Part model, mm, in its own coordinate system. A direction names the side the tool comes from. Coordinates: 2 decimals unless noted, no trailing zeros. Loops run counter-clockwise (first coordinate to the right, second up) from the corner with the lowest first, then second, coordinate; pieces in that order, holes last. Notation, with made-up numbers: M 73,42.5 L 98,42.5 A20 ccw 98,65.5 Z; hole C 80,83.25 d7. An arc over 180 degrees is marked long. Use a Markdown table: item, result. Add a question column.
1) Band-saw the part on C-C (x = -22). List the corners of the cut face in (y, z) (1 decimal).
2) Pull direction X, two halves, no side cores. Call faces 1 (the flat face through (43.815, -4, 0)), 2 (the cylindrical face through (-26.5, -11.3, 0)), 3 (the flat face through (1, -14.288, 0)): released by +X, released by -X, zero draft, split by the parting line, or undercut.
3) Pin check, flat tips, straight feed: pin 1 Ø3 at (x, z) = (18, -2) entering from +Y; pin 2 Ø3 at (y, z) = (-5.5, 1) entering from +X (3 decimals); pin 3 Ø2 at (y, z) = (-4.5, -2) entering from -X (3 decimals). Stop position of each tip, or through.
4) Wall check: probe 1 along X at (y, z) = (-1.5, 2.5) (3 decimals); probe 2 along X at (y, z) = (-9.75, 0); probe 3 along X at (y, z) = (-5, -1.5) (3 decimals). Give the ranges that are in metal, low to high. Write a range as from..to.
5) Tool access for faces 4 (the cylindrical face through (-43.545, -13.333, 0.044)), 5 (the cylindrical face through (-39.25, -5.63, -0.04)), 6 (the flat face through (-40, -10, 1.905)): list every direction of +Z, -Z, +X, -X, +Y, -Y with a clear straight run to the whole face (end or side of a thin tool).
6) Band-saw the part on B-B (x = 0). List the corners of the cut face in (y, z) (1 decimal).
7) Band-saw the part on A-A (y = -1.5). List the corners of the cut face in (x, z) (3 decimals).
Autodesk Inventor part; units mm, degrees
ref_plane "YZ Plane" through (0, 0, 0) normal (1, 0, 0) x (0, 1, 0)
ref_plane "XZ Plane" through (0, 0, 0) normal (0, 1, 0) x (-1, 0, 0)
ref_plane "XY Plane" through (0, 0, 0) normal (0, 0, 1) x (1, 0, 0)
sketch "Sketch1" plane through (0, 0, 0) normal (0, 0, 1) x (1, 0, 0)
  line L0 (-44.45, 14.2875) -> (44.45, 14.2875)
  line L1 (44.45, 14.2875) -> (44.45, -14.2875)
  line L2 (44.45, -14.2875) -> (-44.45, -14.2875)
  line L3 (-44.45, -14.2875) -> (-44.45, 14.2875)
  point P0 (0, 0)
  dimension "d0" = 88.9
  dimension "d1" = 44.45
  dimension "d2" = 14.2875
  dimension "d3" = 28.575
extrude "Extrusion1" add sketch "Sketch1" along normal mid plane 6.35
sketch "Sketch2" plane through (0, 0, 3.175) normal (0, 0, 1) x (1, 0, 0)
  circle A0 centre (-26.2467, 0) radius 11.303
  circle A1 centre (0, 0) radius 11.303
  line L0 (44.45, -14.2875) -> (44.45, 14.2875)
  circle A2 centre (26.2467, 0) radius 11.303
  line L1 (-44.45, 14.2875) -> (-44.45, -14.2875)
  line L2 (-44.45, 0) -> (44.45, 0) construction
  line L3 (44.45, 14.2875) -> (-44.45, 14.2875)
  point P0 (0, 0)
  dimension "d6" = 22.606
  dimension "d9" = 22.606
  dimension "d11" = 22.606
  dimension "d14" = 26.2467
  dimension "d21" = 88.9
  dimension "d22" = 26.2467
  dimension "d50" = 0
sketch "Sketch4" plane through (-44.45, -14.2875, -3.175) normal (-1, 0, 0) x (0, 0, 1)
  line L0 (0, 0) -> (0, 28.575)
  line L1 (6.35, 28.575) -> (6.35, 0)
  line L2 (0, 22.6695) -> (6.35, 22.6695)
  line L3 (6.35, 22.6695) -> (6.35, 5.9055)
  line L4 (6.35, 5.9055) -> (0, 5.9055)
  line L5 (0, 5.9055) -> (0, 22.6695)
  point P0 (3.175, 14.2875)
  dimension "d30" = 8.382
  dimension "d31" = 16.764
extrude "Extrusion3" cut sketch "Sketch4" against normal blind 0.635
mirror "Mirror1" about plane through (0, 0, 0) normal (1, 0, 0) of "Extrusion3"
sketch "Sketch5" plane through (0, 0, 3.175) normal (0, 0, 1) x (1, 0, 0)
  circle A0 centre (0, 9.7155) radius 3.175 construction
  line L0 (44.45, 14.2875) -> (-44.45, 14.2875)
  line L1 (-15.0924, 20.454) -> (43.815, 0) construction
  line L2 (43.815, 8.382) -> (43.815, -8.382)
  circle A1 centre (3.4073, 19.5285) radius 3.175 construction
  circle A2 centre (39.243, 1.5875) radius 3.175 construction
  circle A3 centre (-39.243, 28.8396) radius 3.175 construction
  line L3 (-43.815, 8.382) -> (-43.815, -8.382)
  circle A4 centre (39.878, 9.7155) radius 3.175
  circle A5 centre (-39.878, -9.7155) radius 3.175
  line L4 (44.45, 8.382) -> (44.45, 14.2875)
  line L5 (-44.45, -14.2875) -> (44.45, -14.2875)
  line L6 (-44.45, -14.2875) -> (-44.45, -8.382)
  point P0 (0, 0)
  dimension "d34" = 6.35
  dimension "d35" = 4.572
  dimension "d53" = 6.35
  dimension "d54" = 6.35
  dimension "d55" = 4.572
  dimension "d56" = 4.572
  dimension "d57" = 12.7
  dimension "d58" = 6.35
  dimension "d59" = 6.35
  dimension "d60" = 4.572
  dimension "d61" = 4.572
  dimension "d62" = 4.572
  dimension "d63" = 4.572
extrude "Extrusion4" cut sketch "Sketch5" against normal blind 1.27
sketch "Sketch7" plane through (-44.45, -14.2875, 3.175) normal (0, -1, 0) x (1, 0, 0)
  line L0 (30.48, -14.605) -> (58.42, -14.605)
  line L1 (58.42, -14.605) -> (58.42, 8.255)
  line L2 (58.42, 8.255) -> (30.48, 8.255)
  line L3 (30.48, 8.255) -> (30.48, -14.605)
  point P0 (44.45, -3.175)
  dimension "d39" = 27.94
  dimension "d40" = 22.86
  dimension "d41" = 11.43
  dimension "d42" = 13.97
extrude "Extrusion5" [suppressed]
sketch "Sketch8" plane through (0, 0, -3.175) normal (0, 0, -1) x (-1, 0, 0)
  line L0 (-44.45, 14.2875) -> (44.45, 14.2875)
  line L1 (15.6718, 14.2875) -> (-15.6718, 14.2875)
  line L2 (-15.6718, 14.2875) -> (-15.6718, 52.3875)
  line L3 (-15.6718, 52.3875) -> (15.6718, 52.3875)
  line L4 (15.6718, 52.3875) -> (15.6718, 14.2875)
  point P0 (0, 0)
  dimension "d45" = 31.3436
  dimension "d46" = 38.1
  dimension "d47" = 15.6718
extrude "Extrusion6" add sketch "Sketch8" against normal up to surface (6.35 mm away)
extrude "Extrusion7" cut sketch "Sketch2" against normal blind 25.4
sketch "Sketch9" plane through (-15.6718, 52.3875, -3.175) normal (0, 1, 0) x (1, 0, 0)
  line L0 (-28.7782, -6.35) -> (60.1218, -6.35)
  line L1 (3.1718, -6.35) -> (28.1718, -6.35)
  line L2 (28.1718, -6.35) -> (28.1718, -3.175)
  line L3 (28.1718, -3.175) -> (3.1718, -3.175)
  line L4 (3.1718, -3.175) -> (3.1718, -6.35)
  point P0 (15.6718, -3.175)
  dimension "d64" = 3.175
  dimension "d65" = 25
  dimension "d66" = 12.5
extrude "Extrusion8" cut sketch "Sketch9" against normal blind 0.9
sketch "Sketch13" plane through (0, 0, 3.175) normal (0, 0, 1) x (1, 0, 0)
  line L0 (-15.6718, 52.3875) -> (-12.5, 52.3875)
  line L1 (-12.5, 52.3875) -> (12.5, 52.3875)
  line L2 (12.5, 52.3875) -> (15.6718, 52.3875)
  line L3 (15.6718, 52.3875) -> (15.6718, 14.2875)
  line L4 (-15.6718, 14.2875) -> (-15.6718, 52.3875)
  line L5 (-15.6718, 14.2875) -> (-44.45, 14.2875)
  line L6 (44.45, 14.2875) -> (15.6718, 14.2875)
  line L7 (44.45, 8.382) -> (44.45, 14.2875)
  line L8 (-44.45, 14.2875) -> (-44.45, 8.382)
  line L9 (-44.45, 8.382) -> (-43.815, 8.382)
  line L10 (43.815, 8.382) -> (44.45, 8.382)
  line L11 (-43.815, 8.382) -> (-43.815, 0)
  line L12 (-43.815, 8.382) -> (-43.815, -8.382)
  line L13 (-43.815, 0) -> (43.815, 0)
  line L14 (43.815, 8.382) -> (43.815, -8.382)
  line L15 (43.815, 0) -> (43.815, 8.382)
  point P0 (0, 0)
extrude "Extrusion11" cut sketch "Sketch13" against normal through all
sketch "Sketch14" plane through (-43.815, 0, 3.175) normal (0, 1, 0) x (1, 0, 0)
  line L0 (7.112, 0) -> (0.762, 0)
  line L1 (7.112, 1.27) -> (0.762, 1.27)
  line L2 (6.2653, 6.35) -> (6.2653, 0)
  line L3 (0, 6.35) -> (6.2653, 6.35)
  line L4 (0, 0) -> (0, 6.35)
  line L5 (6.2653, 0) -> (0, 0)
  circle A0 centre (3.1327, 3.81) radius 1.5494
  point P0 (43.815, 3.175)
  dimension "d84" = 3.0988
  dimension "d85" = 6.2653
  dimension "d86" = 5.08
  dimension "d87" = 2.54
  dimension "d88" = 3.1327
extrude "Extrusion12" cut sketch "Sketch14" against normal blind 11.43 contours A0
mirror "Mirror3" about plane through (0, 0, 0) normal (1, 0, 0) of "Extrusion12"
thread "Thread3"
thread "Thread4"
fillet "Fillet1" radius 3.175 2 edges at (44.45, -14.2875, 0) (-44.45, -14.2875, 0)
equation "\"d9\" = d7"
equation "\"d11\" = d9"
equation "\"d22\" = d14"
equation "\"d87\" = 0.5 * d86"
equation "\"d88\" = 0.5 * d85"
equation "\"d7\" = d6"
properties part number "Tube Holder Halve 3" material "Aluminum 6061-AHC"
Entries:
| question | item | result |
|---|---|---|
| 1 | outline | M -14.3,-3.2 L -10.5,-3.2 L -10.5,3.2 L -14.3,3.2 Z |
| 2 | face 1 | released by +X |
| 2 | face 2 | undercut |
| 2 | face 3 | zero draft |
| 3 | pin 1 | y = -5.72 |
| 3 | pin 2 | x = 43.815 |
| 3 | pin 3 | x = -43.815 |
| 4 | probe 1 | -43.815..-37.45, -15.044..-11.203, 11.203..15.044, 37.45..43.815 |
| 4 | probe 2 | -44.45..-42.1, -39.27..-31.96, -20.53..-5.72, 5.72..20.53, 31.96..39.27, 42.1..44.45 |
| 4 | probe 3 | -43.815..-41.968, -39.397..-36.384, -16.11..-10.137, 10.137..16.11, 36.384..39.397, 41.968..43.815 |
| 5 | face 4 | +Z, -Z, -X, -Y |
| 5 | face 5 | +Y |
| 5 | face 6 | +Z |
| 6 | outline | M -14.3,-3.2 L -11.3,-3.2 L -11.3,3.2 L -14.3,3.2 Z |
| 7 | outline | M -43.815,-3.175 L -37.45,-3.175 L -37.45,3.175 L -43.815,3.175 Z; M -15.044,-3.175 L -11.203,-3.175 L -11.203,3.175 L -15.044,3.175 Z; M 11.203,-3.175 L 15.044,-3.175 L 15.044,3.175 L 11.203,3.175 Z; M 37.45,-3.175 L 43.815,-3.175 L 43.815,3.175 L 37.45,3.175 Z; hole C -40.682,-0.635 d3.099; hole C 40.682,-0.635 d3.099 |
